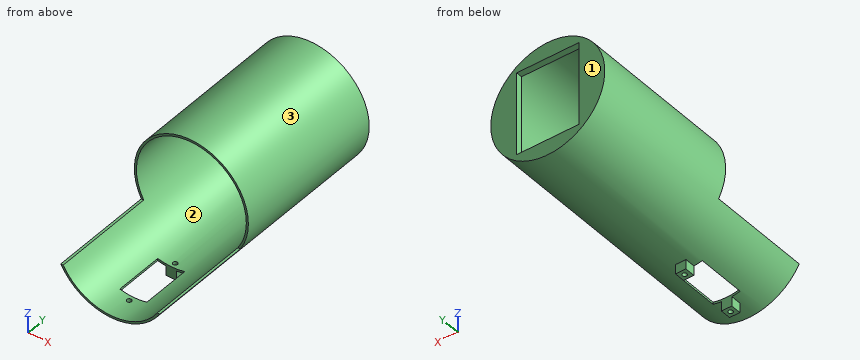
```python
from build123d import *

# Parameters (mm, degrees)
SKETCH_1_R                = 27.5
EXTRUDE_1_DEPTH           = 75
EXTRUDE_1_DEPTH_BACK      = 50
SKETCH_10_W               = 30
SKETCH_10_H               = 40
CUT_EXTRUDE_8_DEPTH       = 45.1
SKETCH_10_2_W             = 30
SKETCH_10_2_H             = 40
CUT_EXTRUDE_9_DEPTH       = 10
CUT_EXTRUDE_9_DEPTH_BACK  = 113
CUT_EXTRUDE_10_DEPTH      = 54
SKETCH_12_R               = 26.5
CUT_EXTRUDE_11_DEPTH      = 72
CUT_EXTRUDE_11_DEPTH_BACK = 55
SKETCH_13_W               = 13
SKETCH_13_H               = 23.5
CUT_EXTRUDE_12_DEPTH      = 54
SKETCH_14_W               = 5
SKETCH_14_H               = 5
EXTRUDE_2_DEPTH           = 1
EXTRUDE_2_DEPTH_BACK      = 4
SKETCH_15_R               = 1.1
CUT_EXTRUDE_13_DEPTH      = 4
CUT_EXTRUDE_13_DEPTH_BACK = 5


with BuildPart() as part:
    # Sketch 1 → Extrude 1 (new body, two sides)
    with BuildSketch(Plane(origin=(0, 0, 0), x_dir=(1, 0, 0), z_dir=(0, 1, 0))) as extrude_1_sk:
        Circle(SKETCH_1_R)
    extrude(amount=EXTRUDE_1_DEPTH)
    extrude(extrude_1_sk.sketch, amount=-EXTRUDE_1_DEPTH_BACK)

    # Sketch 10 → Cut-Extrude 8 (cut)
    with BuildSketch(Plane(origin=(0, 75, 0), x_dir=(1, 0, 0), z_dir=(0, 1, 0))):
        Rectangle(SKETCH_10_W, SKETCH_10_H)
    extrude(amount=-CUT_EXTRUDE_8_DEPTH, mode=Mode.SUBTRACT)

    # Sketch 10_2 → Cut-Extrude 9 (cut, two sides)
    with BuildSketch(Plane(origin=(0, 75, 0), x_dir=(1, 0, 0), z_dir=(0, 1, 0))) as cut_extrude_9_sk:
        Rectangle(SKETCH_10_2_W, SKETCH_10_2_H)
    extrude(amount=CUT_EXTRUDE_9_DEPTH, mode=Mode.SUBTRACT)
    extrude(cut_extrude_9_sk.sketch, amount=-CUT_EXTRUDE_9_DEPTH_BACK, mode=Mode.SUBTRACT)

    # Sketch 11 → Cut-Extrude 10 (cut)
    with BuildSketch(Plane(origin=(0, 0, 0), x_dir=(1, 0, 0), z_dir=(0, 1, 0))):
        with BuildLine():
            Line((23.587956714, 14.137124816), (-24.13203639, 13.186918505))
            ThreePointArc((-24.13203639, 13.186918505), (0.547474823, -27.494549848), (23.587956714, 14.137124816))
        make_face()
    extrude(amount=-CUT_EXTRUDE_10_DEPTH, mode=Mode.SUBTRACT)

    # Sketch 12 → Cut-Extrude 11 (cut, two sides)
    with BuildSketch(Plane(origin=(0, 0, 0), x_dir=(1, 0, 0), z_dir=(0, 1, 0))) as cut_extrude_11_sk:
        Circle(SKETCH_12_R)
    extrude(amount=CUT_EXTRUDE_11_DEPTH, mode=Mode.SUBTRACT)
    extrude(cut_extrude_11_sk.sketch, amount=-CUT_EXTRUDE_11_DEPTH_BACK, mode=Mode.SUBTRACT)

    # Sketch 13 → Cut-Extrude 12 (cut)
    with BuildSketch(Plane.XY):
        with Locations((0, -24.25)):
            Rectangle(SKETCH_13_W, SKETCH_13_H)
    extrude(amount=-CUT_EXTRUDE_12_DEPTH, mode=Mode.SUBTRACT)

    # Sketch 14 → Extrude 2 (add, two sides)
    with BuildSketch(Plane.XY.offset(-28)) as extrude_2_sk:
        with Locations((0, -38.5)):
            Rectangle(SKETCH_14_W, SKETCH_14_H)
        with Locations((0, -10)):
            Rectangle(SKETCH_14_W, SKETCH_14_H)
    extrude(amount=EXTRUDE_2_DEPTH)
    extrude(extrude_2_sk.sketch, amount=-EXTRUDE_2_DEPTH_BACK)

    # Sketch 15 → Cut-Extrude 13 (cut, two sides)
    with BuildSketch(Plane.XY.offset(-28)) as cut_extrude_13_sk:
        with Locations((0, -10)):
            Circle(SKETCH_15_R)
        with Locations((0, -38.5)):
            Circle(SKETCH_15_R)
    extrude(amount=CUT_EXTRUDE_13_DEPTH, mode=Mode.SUBTRACT)
    extrude(cut_extrude_13_sk.sketch, amount=-CUT_EXTRUDE_13_DEPTH_BACK, mode=Mode.SUBTRACT)


solid = part.part
```
Check sheet for the modelled part. Datum: model origin and axes. Units: mm. Face numbers are marked on the shaded views. Coordinates: 2 decimals unless noted, no trailing zeros. Order: outer loops, then holes, each group sorted by start corner. A loop starts at its lowest first (then second) coordinate and runs counter-clockwise, first axis right, second up. Notation, with made-up numbers: (46, 31.5) -> (101, 31.5) arc R13 ccw to (101, 44.5) -> close; hole circle Ø1 at (-6, 39.5). An arc over 180 degrees is marked (long way). Write each question's results on one line, items separated by ' | '. Start each with the question number.
1) Section check C-C (y = 64). Enter the section's corners in (x, z).
2) Depth check by flat-ended pin: pin 1 (1.5 mm diameter, centred on y = 74, z = -1.5, fed in from +X); pin 2 (1.4 mm diameter, centred on x = 1, z = -30, fed in from +Y); pin 3 (1.5 mm diameter, centred on y = -1.5, z = 15.5, fed in from +X); pin 4 (8 mm diameter, centred on x = 21, y = -11.5, fed in from -Z). Enter the tip coordinate at first touch or a pass-through.
3) Section check B-B (y = -14.5). Enter the section's corners in (x, z).
4) Section check A-A (z = 0). Enter the section's corners in (x, y), and give its area (3 significant figures).
5) Material ranges on line 1 along Y through (x, z) = (0, -29); line 2 along X through (y, z) = (17.5, 0), recorded low to high.
6) Section check D-D (z = -17.5). Enter the section's corners in (x, y).
7) Draft check along Z on the marked faces 1, 2 and 3. Enter one of: pulls with the +Z half, pulls with the -Z half, needs draft (parallel to the pull), parting line crosses it, or undercut.
Checked values:
1) outline: circle Ø55 at (0, 0); hole circle Ø53 at (0, 0)
2) pin 1: x = 27.49 | pin 2: y = -7.5 | pin 3: through | pin 4: z = -21.62
3) outline: (-24.13, -13.19) arc R27.5 ccw to (-6.5, -26.72) -> (-6.5, -25.69) arc R26.5 cw to (-22.97, -13.21) -> close; (6.5, -26.72) arc R27.5 ccw to (23.59, -14.14) -> (22.43, -14.11) arc R26.5 cw to (6.5, -25.69) -> close
4) outline: (-27.5, 0) -> (-26.5, 0) -> (-26.5, 72) -> (-15, 72) -> (-15, 75) -> (-27.5, 75) -> close; (15, 72) -> (26.5, 72) -> (26.5, 0) -> (27.5, 0) -> (27.5, 75) -> (15, 75) -> close | area: 219 mm²
5) line 1: -41 to -39.6, -37.4 to -36, -12.5 to -11.1, -8.9 to -7.5 | line 2: -27.5 to -26.5, 26.5 to 27.5
6) outline: (-21.21, -50) -> (-19.9, -50) -> (-19.9, 72) -> (-15, 72) -> (-15, 75) -> (-21.21, 75) -> close; (15, 72) -> (19.9, 72) -> (19.9, -50) -> (21.21, -50) -> (21.21, 75) -> (15, 75) -> close
7) face 1: needs draft | face 2: undercut | face 3: parting line crosses it
